from build123d import *

# Parameters (mm, degrees)
BOSS_EXTRUDE1_DEPTH = 3


with BuildPart() as part:
    # Sketch1 → Boss-Extrude1 (new, symmetric)
    with BuildSketch(Plane.XY):
        Polygon((125, 190), (65, 190), (14.368421053, 42), (125, 42), align=None)
        Polygon((125, 42), (14.368421053, 42), (0, 0), (125, 0), align=None)
    extrude(amount=BOSS_EXTRUDE1_DEPTH, both=True)


solid = part.part
Part model, mm, in its own coordinate system. Coordinates: 2 decimals unless noted, no trailing zeros. Loops run counter-clockwise (first coordinate to the right, second up) from the corner with the lowest first, then second, coordinate; pieces in that order, holes last. Notation, with made-up numbers: (42, 66) - (97, 66) arc R6 cw to (97, 74) - close; hole circle Ø10 at (80.25, 3.5). An arc over 180 degrees is marked (long way). Write each question's results on one line, items separated by ' | '. Start each with the question number.
Q1. Probe line 1 along X through (y, z) = (31.5, -0.5); line 2 along X through (y, z) = (108, -1.25). List the from-to ranges inside material, lowest first.
Q2. Slice it at A-A on z = 0.85. Give the cut face in (x, y), and give its area (3 significant figures).
Q3. Slice it at C-C on x = 37.5. Give the cut face in (y, z), and give its area (3 significant figures).
Q4. Slice it at B-B on y = 38. Give the cut face in (x, z).
Q5. Two-plate mould, pull along Z, no slides. Class faces 1 (the flat face through (125, 94, 0)), 2 (the flat face through (76, 75, -3)), 3 (the flat face through (76, 75, 3)): +Z half, -Z half, draft (parallel to the pull), parting line (faces both ways), or undercut.
Q6. Drop flat-ended pins along their axis: pin 1 Ø2 at (y, z) = (97.5, 1.5) entering from -X; pin 2 Ø1 at (y, z) = (55.5, 0.5) entering from -X. Give the stop position or say it passes through.
Answer:
1) line 1: x = 10.78 to 125 | line 2: x = 36.95 to 125
2) outline: (0, 0) - (125, 0) - (125, 190) - (65, 190) - close | area: 17,600 mm2
3) outline: (0, -3) - (109.62, -3) - (109.62, 3) - (0, 3) - close | area: 658 mm2
4) outline: (13, -3) - (125, -3) - (125, 3) - (13, 3) - close
5) face 1: draft | face 2: -Z half | face 3: +Z half
6) pin 1: stops at x = 33.01 | pin 2: stops at x = 18.82
